The listing builds one solid part. Answer for the finished solid, in the listing's coordinates (mm). Face numbers are marked on the shaded views. A direction names the side the tool comes from. Coordinates: 2 decimals unless noted, no trailing zeros. Loops run counter-clockwise (first coordinate to the right, second up) from the corner with the lowest first, then second, coordinate; pieces in that order, holes last. Notation, with made-up numbers: (51.25, -21) -> (102.25, -21) arc R32 ccw to (102.25, 5) -> close; hole circle Ø2 at (40, -28). An arc over 180 degrees is marked (long way). Answer in a Markdown table with one row per item.
```python
from build123d import *

# Parameters (mm, degrees)
SKETCH1_R           = 8.5
CYLINDER_DEPTH      = 7
SKETCH2_R           = 2.705
LUER_HOLE_DEPTH     = 5
SKETCH3_R           = 1
DOWEL_PINS_DEPTH    = 2.5
SKETCH4_R           = 1
SCREW_HOLES_DEPTH   = 14.910427743
FILLET_DOWEL_PINS_R = 0.5


with BuildPart() as part:
    # Sketch1 → Cylinder (new body)
    with BuildSketch(Plane(origin=(0, 0, 0), x_dir=(1, 0, 0), z_dir=(0, 1, 0))):
        with Locations(Location((0, 0, 0), (0, 0, 270))):
            Circle(SKETCH1_R)
    extrude(amount=CYLINDER_DEPTH)

    # Sketch2 → Luer Hole (cut)
    with BuildSketch(Plane(origin=(0, 7, 0), x_dir=(1, 0, 0), z_dir=(0, 1, 0))):
        with Locations(Location((0, 0, 0), (0, 0, 270))):
            Circle(SKETCH2_R)
    extrude(amount=-LUER_HOLE_DEPTH, mode=Mode.SUBTRACT)

    # Sketch3 → Dowel Pins (add)
    with BuildSketch(Plane.XZ):
        with Locations(Location((-1.08530111, 6.155048456, 0), (0, 0, 90))):
            Circle(SKETCH3_R)
        with Locations(Location((5.87307888, -2.137625896, 0), (0, 0, 90))):
            Circle(SKETCH3_R)
    extrude(amount=DOWEL_PINS_DEPTH)

    # Sketch4 → Screw Holes (cut, through all)
    with BuildSketch(Plane.XZ):
        with Locations(Location((-6.226216863, -0.544723392, 0), (0, 0, 270))):
            Circle(SKETCH4_R)
        with Locations(Location((2.641364136, 5.664423669, 0), (0, 0, 270))):
            Circle(SKETCH4_R)
        with Locations(Location((3.584852727, -5.119700277, 0), (0, 0, 270))):
            Circle(SKETCH4_R)
    extrude(amount=-SCREW_HOLES_DEPTH, mode=Mode.SUBTRACT)

    # Fillet Dowel Pins
    fillet_dowel_pins_edges = [part.edges().sort_by_distance(p)[0] for p in [
        (-1.08530111, -2.5, 5.155048456),
        (5.87307888, -2.5, -3.137625896),
    ]]
    fillet(fillet_dowel_pins_edges, radius=FILLET_DOWEL_PINS_R)


solid = part.part
```
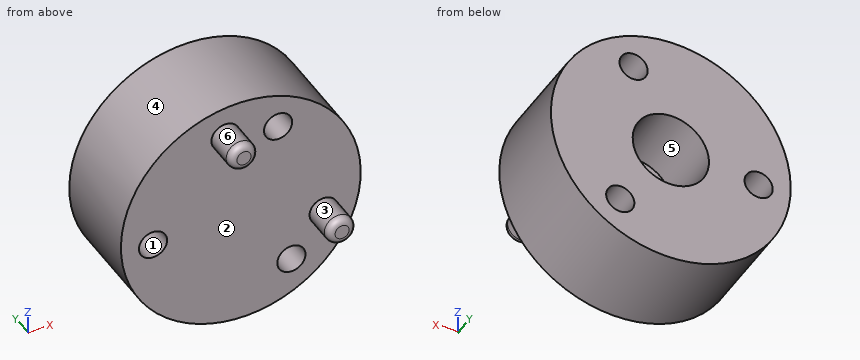
Item 1: Find the intervals of material crossed by probe 1 along X at (y, z) = (5.3, 0) (3 decimals); probe 2 along Z at (x, y) = (3.25, 3.5); probe 3 along Y at (x, z) = (0.5, -5), in increasing order.
Findings below:
| item | result |
|---|---|
| probe 1 | x = -8.5 to -7.065, -5.388 to -2.705, 2.705 to 8.5 |
| probe 2 | z = -7.85 to -6.06, -4.18 to 4.87, 6.46 to 7.85 |
| probe 3 | y = 0 to 7 |
Item 2: Determine the mould class of the marked faces 1, 2 and 3 for opening direction Z: +Z half, -Z half, draft (parallel to the pull), parting line (faces both ways), or undercut.
Findings below:
| item | result |
|---|---|
| face 1 | undercut |
| face 2 | draft |
| face 3 | parting line |
Item 3: A cutting plane is placed at B-B, the plane x = 1.25. Determine the outline of the cut face in (y, z), plus the area to 3 significant figures.
Findings below:
| item | result |
|---|---|
| outline | (0, -8.41) -> (7, -8.41) -> (7, -2.4) -> (2, -2.4) -> (2, 2.4) -> (7, 2.4) -> (7, 8.41) -> (0, 8.41) -> close |
| area | 93.7 mm2 |
Item 4: A tool of negligible diameter and unlimited length cuts with its end or side. For the marked faces 4, 5 and 6, from which of +Z, -Z, +X, -X, +Y, -Y can it reach the whole face along a straight path? Write none if from no direction.
Findings below:
| item | result |
|---|---|
| face 4 | +Y, -Y |
| face 5 | +Y |
| face 6 | -Y |
Item 5: A cutting plane is placed at A-A, the plane z = 0. Determine the outline of the cut face in (x, y) (3 decimals), plus the area to 3 significant figures.
Findings below:
| item | result |
|---|---|
| outline | (-8.5, 0) -> (-7.065, 0) -> (-7.065, 7) -> (-8.5, 7) -> close; (-5.388, 0) -> (8.5, 0) -> (8.5, 7) -> (2.705, 7) -> (2.705, 2) -> (-2.705, 2) -> (-2.705, 7) -> (-5.388, 7) -> close |
| area | 80.2 mm2 |
Item 6: A cutting plane is placed at C-C, the plane y = 0.5. Determine the outline of the cut face in (x, z), plus the area to 3 significant figures.
Findings below:
| item | result |
|---|---|
| outline | circle Ø17 at (0, 0); hole circle Ø2 at (-6.23, -0.54); hole circle Ø2 at (2.64, 5.66); hole circle Ø2 at (3.58, -5.12) |
| area | 218 mm2 |
Item 7: A cutting plane is placed at D-D, the plane y = 3.5. Determine the outline of the cut face in (x, z) (3 decimals), plus the area to 3 significant figures.
Findings below:
| item | result |
|---|---|
| outline | circle Ø17 at (0, 0); hole circle Ø2 at (-6.226, -0.545); hole circle Ø5.41 at (0, 0); hole circle Ø2 at (2.641, 5.664); hole circle Ø2 at (3.585, -5.12) |
| area | 195 mm2 |
Item 8: Flat-ended cylindrical pins translate along their axes: pin 1 Ø8 at (x, z) = (3.5, -1) entering from -Y; pin 2 Ø4 at (x, y) = (-3, 1) entering from +Z; pin 3 Ø7 at (x, z) = (0, 0) entering from -Y; pin 4 Ø4 at (y, z) = (2.5, 6) entering from -X. Find the tip coordinate at first contact, or state that the pin passes through.
Findings below:
| item | result |
|---|---|
| pin 1 | stops at y = -2.5 |
| pin 2 | stops at z = 8.44 |
| pin 3 | stops at y = 0 |
| pin 4 | stops at x = -7.5 |
